Check sheet for the drawn part. Datum: minimum x, y, z corner. Units: mm. A direction names the side the tool comes from. Coordinates: 2 decimals unless noted, no trailing zeros. Order: outer loops, then holes, each group sorted by start corner. A loop starts at its lowest first (then second) coordinate and runs counter-clockwise, first axis right, second up.
Q1. Cross-section at D-D, the plane z = 9.25. Record the boundary of the cut face in (x, y).
Q2. Cross-section at C-C, the plane z = 5. Record the boundary of the cut face in (x, y).
Q3. Thickness scan on line 1 (X direction, y = 2, z = 5); line 2 (X direction, y = 2.25, z = 1); line 3 (Y direction, x = 29.5, z = 8.75). Record the ranges inside material, lowest first.
Q4. Cross-section at A-A, the plane x = 2.5. Record the boundary of the cut face in (y, z), and give its area (3 significant figures).
Q5. Cross-section at B-B, the plane y = 6. Record the boundary of the cut face in (x, z), and give its area (3 significant figures).
Q6. Set-up check for the marked faces 1, 2, 3 and 4: record each of +Z, -Z, +X, -X, +Y, -Y from which the full face is reachable in a straight line by a thin tool's end or side.
Q7. Draft check along X on the marked faces 5, 6 and 7. Enter one of: pulls with the +X half, pulls with the -X half, needs draft (parallel to the pull), parting line crosses it, or undercut.
Q8. Depth check by flat-ended pin: P1, Ø4, axis at x = 2, z = 6.5, coming from the +Y side; P2, Ø5, axis at x = 16, z = 5.5, coming from the -Y side; P3, Ø3.5, axis at y = 7, z = 7, coming from the -X side. Enter the tip coordinate at first touch or a pass-through.
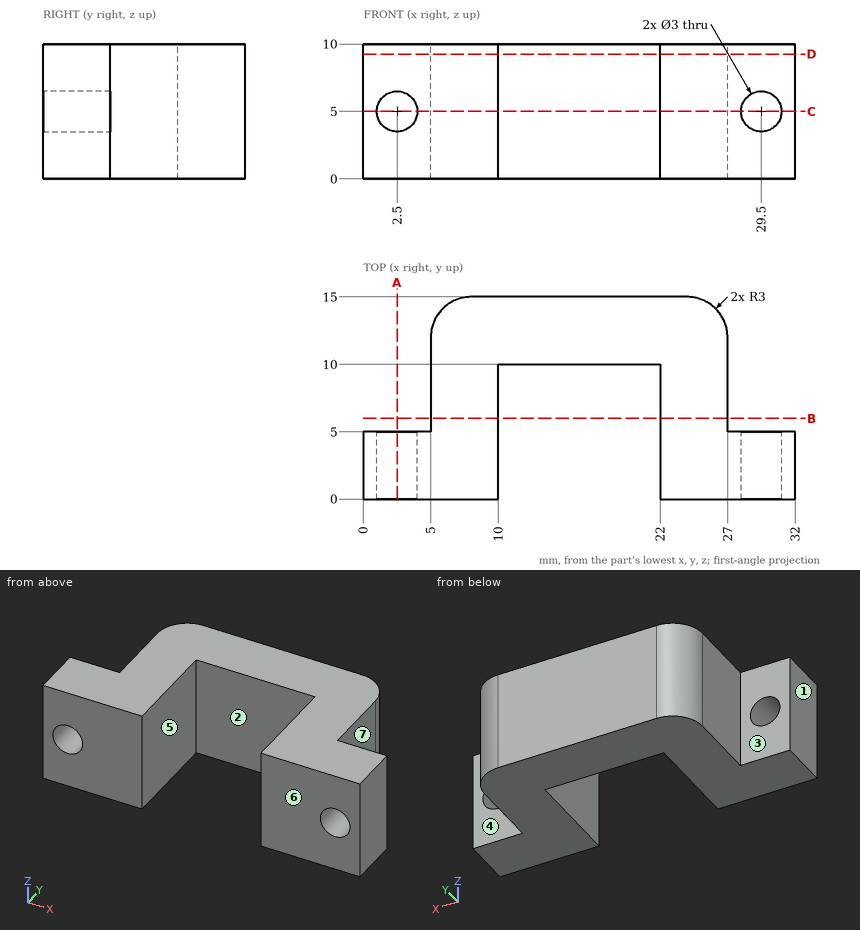
Check values:
1. outline: (0, 0) - (10, 0) - (10, 10) - (22, 10) - (22, 0) - (32, 0) - (32, 5) - (27, 5) - (27, 12) arc R3 ccw to (24, 15) - (8, 15) arc R3 ccw to (5, 12) - (5, 5) - (0, 5) - close
2. outline: (0, 0) - (1, 0) - (1, 5) - (0, 5) - close; (4, 0) - (10, 0) - (10, 10) - (22, 10) - (22, 0) - (28, 0) - (28, 5) - (27, 5) - (27, 12) arc R3 ccw to (24, 15) - (8, 15) arc R3 ccw to (5, 12) - (5, 5) - (4, 5) - close; (31, 0) - (32, 0) - (32, 5) - (31, 5) - close
3. line 1: x = 0 to 1, 4 to 10, 22 to 28, 31 to 32
3. line 2: x = 0 to 10, 22 to 32
3. line 3: y = 0 to 5
4. outline: (0, 0) - (5, 0) - (5, 3.5) - (0, 3.5) - close; (0, 6.5) - (5, 6.5) - (5, 10) - (0, 10) - close
4. area: 35.0 mm2
5. outline: (5, 0) - (10, 0) - (10, 10) - (5, 10) - close; (22, 0) - (27, 0) - (27, 10) - (22, 10) - close
5. area: 100 mm2
6. face 1: +Z, -Z, -X, +Y, -Y
6. face 2: +Z, -Z, -Y
6. face 3: +Z, -Z, -X, +Y
6. face 4: +Z, -Z, +X, +Y
7. face 5: undercut
7. face 6: needs draft
7. face 7: pulls with the +X half
8. P1: stops at y = 5
8. P2: stops at y = 10
8. P3: stops at x = 5
